```python
from build123d import *

# Parameters (mm, degrees)
SKETCH1_W               = 76.2
SKETCH1_H               = 76.2
SKETCH1_R               = 3.175
BOSS_EXTRUDE1_DEPTH     = 3.175
F_1_4_28_TAPPED_HOLE3_D = 5.4102


with BuildPart() as part:
    # Sketch1 → Boss-Extrude1 (new body)
    with BuildSketch(Plane.XY):
        with Locations((49.8593053, 265.676157482)):
            Rectangle(SKETCH1_W, SKETCH1_H)
        with Locations((25.4, 235.857142857)):
            Circle(SKETCH1_R, mode=Mode.SUBTRACT)
        with Locations((25.4, 294.821428571)):
            Circle(SKETCH1_R, mode=Mode.SUBTRACT)
        with Locations((76.2, 235.857142857)):
            Circle(SKETCH1_R, mode=Mode.SUBTRACT)
        with Locations((76.2, 294.821428571)):
            Circle(SKETCH1_R, mode=Mode.SUBTRACT)
    extrude(amount=BOSS_EXTRUDE1_DEPTH)

    # 1/4-28 Tapped Hole3 (through all)
    with Locations(Plane.XY.offset(3.175)):
        with Locations((55.4677219, 287.273383219)):
            Hole(F_1_4_28_TAPPED_HOLE3_D / 2)


solid = part.part
```
Input: part model. Units: mm. Frame: model coordinates. Coordinates: 2 decimals unless noted, no trailing zeros. Loops run counter-clockwise (first coordinate to the right, second up) from the corner with the lowest first, then second, coordinate; pieces in that order, holes last. Notation, with made-up numbers: M 35.5,86.25 L 92.5,86.25 A28 cw 92.5,123.25 Z; hole C -15.75,-22 d5. An arc over 180 degrees is marked long. Use a Markdown table: item, result. Add a question column.
1) Pin query (flat end, axial travel): P1, Ø4, axis at x = 21.5, y = 290, coming from the -Z side; P2, Ø4, axis at x = 25.4, y = 235.86, coming from the -Z side. Return the tip coordinate at first contact, or that it passes through.
2) Section B-B, the plane z = 2.1. Return the cut outline in (x, y) (3 decimals), plus the area to 3 significant figures.
3) Line query: L1, parallel to Y at x = 25.4, z = 0.7; L2, parallel to Y at x = 75.5, z = 2.3; L3, parallel to Y at x = 54.5, z = 1.3. Output: solid intervals per line, ascending. Write a range as from..to.
4) Draft query along X for faces 1 (the flat face through (49, 303.776, 2)), 2 (the flat face through (87.959, 265, 2)), 3 (the cylindrical face through (77.907, 297.499, 1.565)). Return one class per face: +X half, -X half, draft (parallel to the pull), parting line (faces both ways), or undercut.
5) Section A-A, the plane x = 76.2. Return the cut outline in (y, z) (3 decimals).
Answer below:
| question | item | result |
|---|---|---|
| 1 | P1 | z = 0 |
| 1 | P2 | through |
| 2 | outline | M 11.759,227.576 L 87.959,227.576 L 87.959,303.776 L 11.759,303.776 Z; hole C 25.4,235.857 d6.35; hole C 25.4,294.821 d6.35; hole C 55.468,287.273 d5.41; hole C 76.2,235.857 d6.35; hole C 76.2,294.821 d6.35 |
| 2 | area | 5,660 mm2 |
| 3 | L1 | 227.58..232.68, 239.03..291.65, 298..303.78 |
| 3 | L2 | 227.58..232.76, 238.95..291.72, 297.92..303.78 |
| 3 | L3 | 227.58..284.75, 289.8..303.78 |
| 4 | face 1 | draft |
| 4 | face 2 | +X half |
| 4 | face 3 | undercut |
| 5 | outline | M 227.576,0 L 232.682,0 L 232.682,3.175 L 227.576,3.175 Z; M 239.032,0 L 291.646,0 L 291.646,3.175 L 239.032,3.175 Z; M 297.996,0 L 303.776,0 L 303.776,3.175 L 297.996,3.175 Z |
